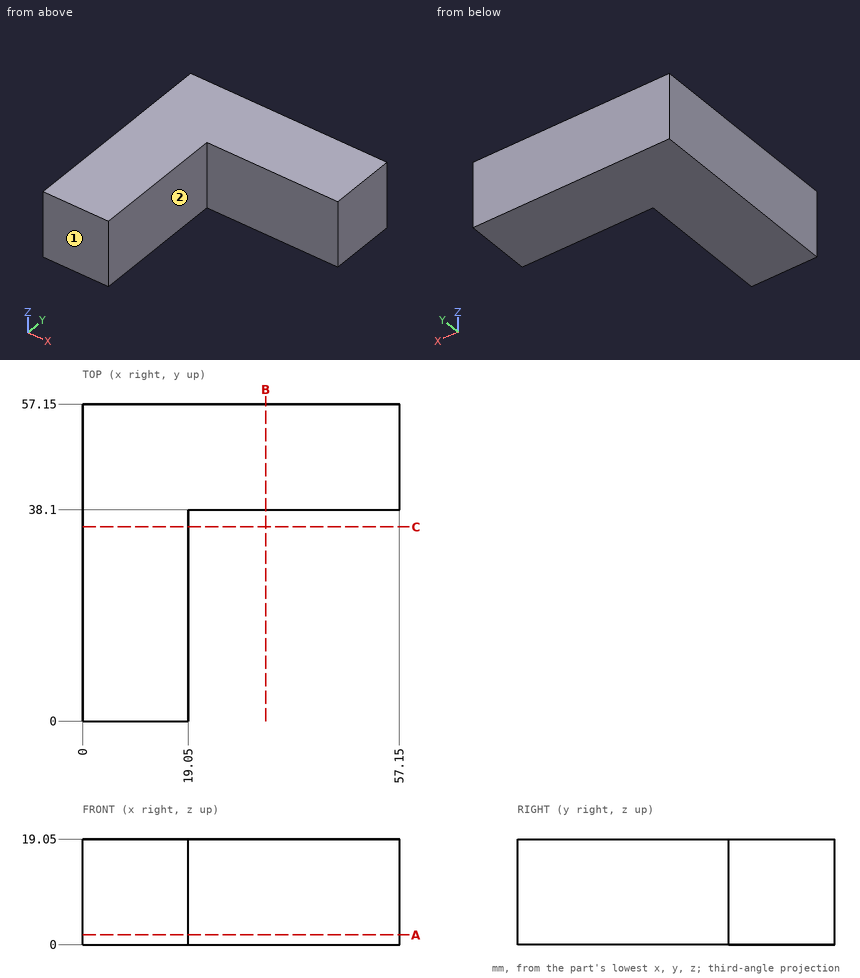
Design review of the part shown in the three views and the two pictorial views. Dimensions are in mm from the part's minimum x, y and z. A direction names the side the tool comes from. Round coordinates to 2 decimals unless told otherwise and drop trailing zeros. Order: outer loops, then holes, each group sorted by start corner. A loop starts at its lowest first (then second) coordinate and runs counter-clockwise, first axis right, second up. Notation, with made-up numbers: (83, 3) -> (137, 3) arc R15 cw to (137, 9) -> close; hole circle Ø4 at (52.5, 60.5). An arc over 180 degrees is marked (long way). Write item = value, one per line. Start each with the question number.
1) Insertion check: pin 1 (4 mm diameter, centred on y = 30.5, z = 15.5, fed in from -X); pin 2 (10 mm diameter, centred on x = 24.5, z = 11.5, fed in from -Y). Each pin has a flat end and moves straight along its axis. Give the tip position at first contact, or say it passes through.
2) Take a section at B-B on x = 33. State the section outline as (y, z) points, plus the area to 3 significant figures.
3) To check wall thickness, follow line 1 (X direction, y = 16.5, z = 14); line 2 (Y direction, x = 53, z = 4). State the ranges of each line that lie inside material, in increasing order. Write a range as from..to.
4) Tool access review of the marked faces 1 and 2: name each direction out of +Z, -Z, +X, -X, +Y, -Y from which nothing blocks a thin tool from reaching the whole face with its end or side.
5) Take a section at A-A on z = 1.75. State the section outline as (x, y) points, plus the area to 3 significant figures.
6) Take a section at C-C on y = 35. State the section outline as (x, z) points, plus the area to 3 significant figures.
Verdict:
q1.pin_1 = 0
q1.pin_2 = 38.1
q2.outline = (38.1, 0) -> (57.15, 0) -> (57.15, 19.05) -> (38.1, 19.05) -> close
q2.area = 363 mm2
q3.line_1 = 0..19.05
q3.line_2 = 38.1..57.15
q4.face_1 = +Z, -Z, +X, -X, -Y
q4.face_2 = +Z, -Z, +X, -Y
q5.outline = (0, 0) -> (19.05, 0) -> (19.05, 38.1) -> (57.15, 38.1) -> (57.15, 57.15) -> (0, 57.15) -> close
q5.area = 1,810 mm2
q6.outline = (0, 0) -> (19.05, 0) -> (19.05, 19.05) -> (0, 19.05) -> close
q6.area = 363 mm2
